Design review of the part shown in the three views and the two pictorial views. Dimensions are in mm from the part's minimum x, y and z. Give positions to 0.01 mm unless a question says otherwise; leave off trailing zeros. Loops run counter-clockwise (first coordinate to the right, second up) from the corner with the lowest first, then second, coordinate; pieces in that order, holes last. Notation, with made-up numbers: (79.5, -23) -> (137.5, -23) arc R14 ccw to (137.5, -18) -> close; hole circle Ø6 at (71.5, 44.25). An arc over 180 degrees is marked (long way). One line per question, with ' | ' between items. Start each with the question number.
(1) Consider section A-A (y = 16.5). Write out the cut boundary in (x, z).
(2) Insertion check: P1, Ø8, axis at y = 15, z = 153, coming from the -X side. The pin has a flat end and moves straight along its axis. Give the tip position at first contact, or say it passes through.
(3) Consider section B-B (x = 5.25). Write out the cut boundary in (y, z) (3 decimals).
(4) Wall thickness on probe 1 along Z at (x, y) = (6, 11.5); probe 2 along Z at (x, y) = (5.25, 19.5); probe 3 along Z at (x, y) = (3.5, 8.5): over which ranges is each line inside the solid? List them lowest first.
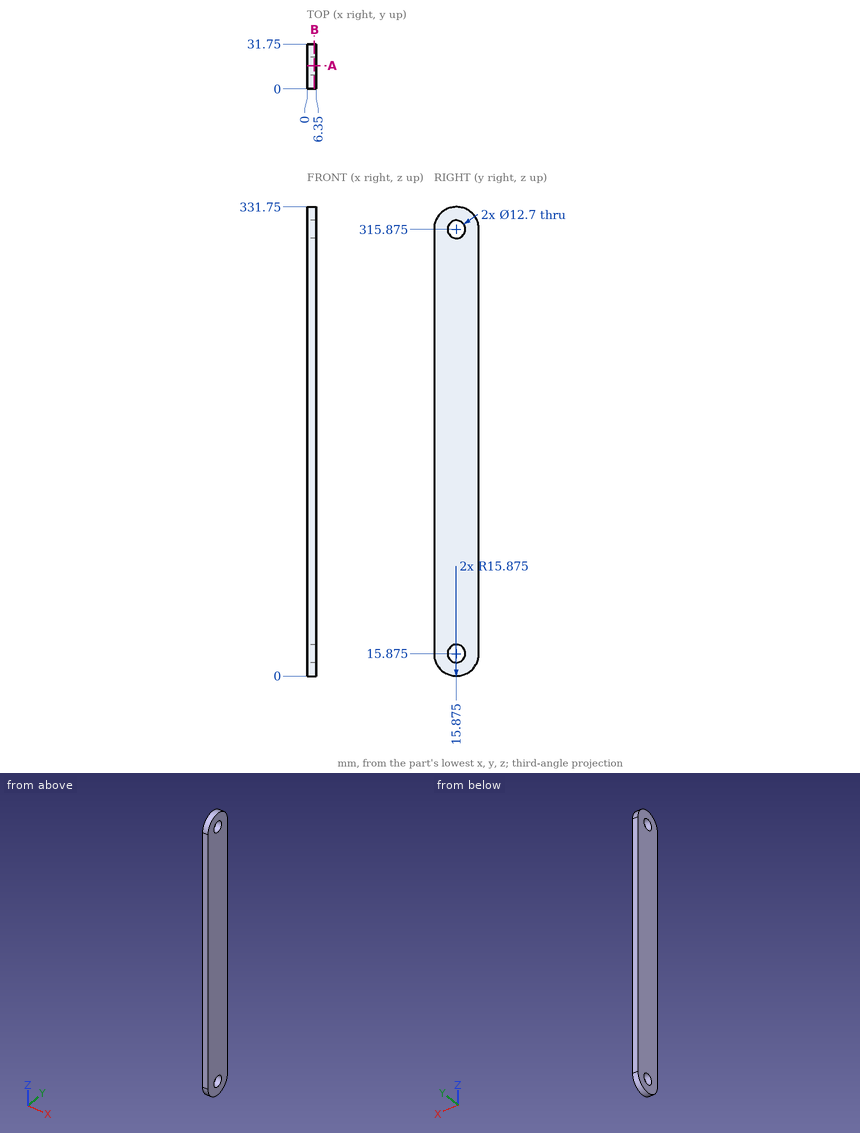
A:
1) outline: (0, 0.01) -> (6.35, 0.01) -> (6.35, 9.56) -> (0, 9.56) -> close; (0, 22.19) -> (6.35, 22.19) -> (6.35, 309.56) -> (0, 309.56) -> close; (0, 322.19) -> (6.35, 322.19) -> (6.35, 331.74) -> (0, 331.74) -> close
2) P1: stops at x = 0
3) outline: (0, 15.875) arc R15.875 ccw to (31.75, 15.875) -> (31.75, 315.875) arc R15.875 ccw to (0, 315.875) -> close; hole circle Ø12.7 at (15.875, 15.875); hole circle Ø12.7 at (15.875, 315.875)
4) probe 1: z = 0.61 to 11.27, 20.48 to 311.27, 320.48 to 331.14 | probe 2: z = 0.42 to 10.66, 21.09 to 310.66, 321.09 to 331.33 | probe 3: z = 1.82 to 329.93
